from build123d import *

# Parameters (mm, degrees)
SKETCH1_R           = 1.05
SKETCH1_W           = 12.2
SKETCH1_H           = 10.2
BOSS_EXTRUDE1_DEPTH = 2
SKETCH2_W           = 16.2
SKETCH2_H           = 14.2
SKETCH2_W_2         = 12.2
SKETCH2_H_2         = 10.2
BOSS_EXTRUDE2_DEPTH = 7
SKETCH4_W           = 16.2
SKETCH4_H           = 14.2
SKETCH4_R           = 2
BOSS_EXTRUDE3_DEPTH = 1
FILLET1_R           = 1.5
CUT_EXTRUDE1_DEPTH  = 7
FILLET2_R           = 2
FILLET3_R           = 1
CHAMFER2_SIZE       = 1
SKETCH6_R           = 0.8
CUT_EXTRUDE2_DEPTH  = 1
CHAMFER3_SIZE       = 0.8


with BuildPart() as part:
    # Sketch1 → Boss-Extrude1 (new body)
    with BuildSketch(Plane(origin=(0, 0, 0), x_dir=(1, 0, 0), z_dir=(0, 1, 0))):
        with BuildLine():
            Line((-16.83443407, -1.126269728), (-13.645952788, -9.15058198))
            ThreePointArc((-13.645952788, -9.15058198), (-12.480190316, -10.602941562), (-10.7, -11.15))
            Line((-10.7, -11.15), (3.9, -11.15))
            Line((3.9, -11.15), (3.9, 0.2))
            Line((3.9, 0.2), (3.9, 14.4))
            Line((3.9, 14.4), (-12.3, 14.4))
            Line((-12.3, 14.4), (-12.3, 3.05))
            Line((-12.3, 3.05), (-14, 3.05))
            ThreePointArc((-14, 3.05), (-16.523650399, 1.712801408), (-16.83443407, -1.126269728))
        make_face()
        with Locations(Location((-14, 0, 0), (0, 0, 270))):
            Circle(SKETCH1_R, mode=Mode.SUBTRACT)
        with Locations(Location((0, -9.3, 0), (0, 0, 270))):
            Circle(SKETCH1_R, mode=Mode.SUBTRACT)
        with Locations(Location((-10.7, -7.98, 0), (0, 0, 270))):
            Circle(SKETCH1_R, mode=Mode.SUBTRACT)
        with Locations((-4.2, 7.3)):
            Rectangle(SKETCH1_W, SKETCH1_H, mode=Mode.SUBTRACT)
    extrude(amount=BOSS_EXTRUDE1_DEPTH)

    # Sketch2 → Boss-Extrude2 (add)
    with BuildSketch(Plane.XZ):
        with Locations((-4.2, -7.3)):
            Rectangle(SKETCH2_W, SKETCH2_H)
        with Locations((-4.2, -7.3)):
            Rectangle(SKETCH2_W_2, SKETCH2_H_2, mode=Mode.SUBTRACT)
    extrude(amount=BOSS_EXTRUDE2_DEPTH)

    # Sketch4 → Boss-Extrude3 (add)
    with BuildSketch(Plane.XZ.offset(7)):
        with Locations((-4.2, -7.3)):
            Rectangle(SKETCH4_W, SKETCH4_H)
        with Locations(Location((-4.2, -7.3, 0), (0, 0, 270))):
            Circle(SKETCH4_R, mode=Mode.SUBTRACT)
    extrude(amount=-BOSS_EXTRUDE3_DEPTH)

    # Fillet1
    fillet1_edges = [part.edges().sort_by_distance(p)[0] for p in [
        (-12.3, -2.5, -14.4),
        (3.9, -2.5, -14.4),
        (3.9, 1, 11.15),
        (-12.3, 1, -3.05),
        (3.9, -3.5, -0.2),
        (-12.3, -3.5, -0.2),
    ]]
    fillet(fillet1_edges, radius=FILLET1_R)

    # Sketch5 → Cut-Extrude1 (cut)
    with BuildSketch(Plane.XZ.offset(7)):
        Polygon((-12.3, -2.375849406), (-12.3, -0.2), (-9.840369616, -0.2), align=None)
    extrude(amount=-CUT_EXTRUDE1_DEPTH, mode=Mode.SUBTRACT)

    # Fillet2
    fillet2_edges = [part.edges().sort_by_distance(p)[0] for p in [
        (-12.3, -3.5, -2.375849406),
        (-9.840369616, -3.5, -0.2),
    ]]
    fillet(fillet2_edges, radius=FILLET2_R)

    # Fillet3
    fillet3_edges = [part.edges().sort_by_distance(p)[0] for p in [
        (1.9, -2, -2.2),
        (1.9, -2, -12.4),
        (-10.3, -2, -12.4),
        (-10.3, -2, -2.2),
    ]]
    fillet(fillet3_edges, radius=FILLET3_R)

    # Chamfer2
    # the kernel refuses this chamfer: 1 mm, written as the material it takes off along each edge
    with BuildSketch(Plane(origin=(-14, 2, 0), x_dir=(0, 0, 1), z_dir=(-1, 0, 0))) as chamfer2_piece_1:
        Polygon((1.05 + CHAMFER2_SIZE, 0), (1.05, -CHAMFER2_SIZE), (1.05, 0), align=None)
    revolve(axis=Axis((-14, 2, 0), (0, 1, 0)), mode=Mode.SUBTRACT)
    with BuildSketch(Plane(origin=(0, 2, 9.3), x_dir=(0, 0, 1), z_dir=(-1, 0, 0))) as chamfer2_piece_2:
        Polygon((1.05 + CHAMFER2_SIZE, 0), (1.05, -CHAMFER2_SIZE), (1.05, 0), align=None)
    revolve(axis=Axis((0, 2, 9.3), (0, 1, 0)), mode=Mode.SUBTRACT)
    with BuildSketch(Plane(origin=(-10.7, 2, 7.98), x_dir=(0, 0, 1), z_dir=(-1, 0, 0))) as chamfer2_piece_3:
        Polygon((1.05 + CHAMFER2_SIZE, 0), (1.05, -CHAMFER2_SIZE), (1.05, 0), align=None)
    revolve(axis=Axis((-10.7, 2, 7.98), (0, 1, 0)), mode=Mode.SUBTRACT)

    # Sketch6 → Cut-Extrude2 (cut)
    with BuildSketch(Plane.XZ.offset(7)):
        with Locations(Location((-9.2, -7.3, 0), (0, 0, 270))):
            Circle(SKETCH6_R)
        with Locations(Location((0.8, -7.3, 0), (0, 0, 270))):
            Circle(SKETCH6_R)
    extrude(amount=-CUT_EXTRUDE2_DEPTH, mode=Mode.SUBTRACT)

    # Chamfer3
    chamfer3_edges = [part.edges().sort_by_distance(p)[0] for p in [
        (-9.2, -7, -6.5),
        (0.8, -7, -6.5),
    ]]
    chamfer(chamfer3_edges, length=CHAMFER3_SIZE)


solid = part.part
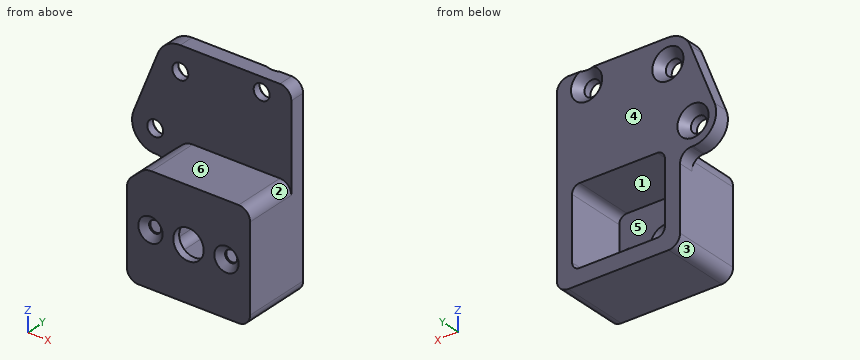
Here's how the part is built. I have some questions about the finished solid (model axes, mm). Face numbers are marked on the shaded views. A direction names the side the tool comes from. Round coordinates to 2 decimals unless told otherwise and drop trailing zeros. Loops run counter-clockwise (first coordinate to the right, second up) from the corner with the lowest first, then second, coordinate; pieces in that order, holes last. Notation, with made-up numbers: M 85,50 L 129,50 A26 cw 129,67 Z; hole C 62,81.5 d10. An arc over 180 degrees is marked long. Write each question's results on one line, items separated by ' | '. Start each with the question number.
(1) Will these pins go through, and if not, where does the flat tip stop? P1, Ø8, axis at x = -5.5, z = 8, coming from the -Y side; P2, Ø4, axis at y = 0, z = -8.5, coming from the -X side; P3, Ø4, axis at x = 0.5, z = -3.5, coming from the +Y side; P4, Ø5, axis at x = -7, z = -7.5, coming from the +Y side.
(2) If I drill on probe 1 along X at (y, z) = (-6.1, -7.3); probe 2 along Z at (x, y) = (-2.25, -2.25); probe 3 along X at (y, z) = (-2, -3.25), over which ranges is the centre line in solid material (lowest first)? Write a range as from..to.
(3) I want a section at A-A (y = -2). Please give me the cut outline in (x, z).
(4) On a 3-axis mill with a long thin cutter (end or side, diameter ignored), from which of +Z, -Z, +X, -X, +Y, -Y can I reach the whole of each face in a straight line? I mean the marked faces 4, 5 and 6. Say none if no direction works.
(5) I want a section at B-B (x = -4.2). Please give me the cut outline in (y, z), then the cut area to 3 significant figures.
(6) Thinking about a two-plate mould opening in X: for the marked faces 1, 2 and 3, which applies, pulls with the +X half, pulls with the -X half, needs draft (parallel to the pull), parting line crosses it, or undercut?
(7) I want a section at D-D (x = -6.75). Please give me the cut outline in (y, z).
(8) I want a section at C-C (z = -11). Please give me the cut outline in (x, y).
Solved:
1) P1: stops at y = 0 | P2: stops at x = -12.3 | P3: stops at y = 2 | P4: stops at y = -6
2) probe 1: x = -12.3..-10, -8.4..-6.2, -2.2..0, 1.6..3.9 | probe 2: z = -14.4..-12.4, -2.2..-0.2 | probe 3: x = -12.3..-10.3, 1.9..3.9
3) outline: M -12.3,-12.9 A1.5 ccw -10.8,-14.4 L 2.4,-14.4 A1.5 ccw 3.9,-12.9 L 3.9,-1.7 A1.5 ccw 2.4,-0.2 L -9.08,-0.2 A2 ccw -10.41,-0.7 L -11.63,-1.78 A2 ccw -12.3,-3.28 Z; hole M -10.3,-11.4 A1 ccw -9.3,-12.4 L 0.9,-12.4 A1 ccw 1.9,-11.4 L 1.9,-3.2 A1 ccw 0.9,-2.2 L -9.3,-2.2 A1 ccw -10.3,-3.2 Z
4) face 4: +Z, -Z, +X, -X, +Y | face 5: +Y | face 6: +Z, +X, -X, -Y
5) outline: M -7,-14.4 L 2,-14.4 L 2,-12.4 L -6,-12.4 L -6,-9.3 L -7,-9.3 Z; M -7,-5.3 L -6,-5.3 L -6,-2.2 L 2,-2.2 L 2,11.15 L 0,11.15 L 0,-0.2 L -7,-0.2 Z | area: 64.9 mm²
6) face 1: undercut | face 2: pulls with the +X half | face 3: pulls with the -X half
7) outline: M -7,-14.4 L 2,-14.4 L 2,-12.4 L -6,-12.4 L -6,-2.2 L 2,-2.2 L 2,11.15 L 0,11.15 L 0,-0.2 L -7,-0.2 Z
8) outline: M -12.3,-7 L 3.9,-7 L 3.9,2 L 1.9,2 L 1.9,-6 L -10.3,-6 L -10.3,2 L -12.3,2 Z
